from build123d import *

# Parameters (mm, degrees)
F0_R     = 6.35
F1_DEPTH = 12.7
F3_DEPTH = 22.225
F4_W     = 50.8
F4_H     = 25.4
F5_DEPTH = 44.45
F6_R     = 3.175
F7_DEPTH = 25.4


with BuildPart() as f1:
    # F0 (on Front) → F1 (new body)
    with BuildSketch(Plane.XZ):
        with BuildLine():
            Line((64.422844, 12.7), (-62.577156, 12.7))
            ThreePointArc((-62.577156, 12.7), (-75.277156, 0), (-62.577156, -12.7))
            Line((-62.577156, -12.7), (64.422844, -12.7))
            ThreePointArc((64.422844, -12.7), (77.122844, 0), (64.422844, 12.7))
        make_face()
        with Locations((-62.577156, 0)):
            Circle(F0_R, mode=Mode.SUBTRACT)
        with Locations((64.422844, 0)):
            Circle(F0_R, mode=Mode.SUBTRACT)
    extrude(amount=F1_DEPTH)

    # F2 (on Top) → F3 (join, symmetric)
    with BuildSketch(Plane.XY):
        with BuildLine():
            Line((44.45, 0), (-44.45, 0))
            ThreePointArc((-44.45, 0), (0, -44.45), (44.45, 0))
        make_face()
    extrude(amount=F3_DEPTH, both=True)

    # F4 (on face) → F5 (cut)
    with BuildSketch(Plane(origin=(0, 0, -22.225), x_dir=(1, 0, 0), z_dir=(0, 0, -1))):
        with Locations((0, 12.7)):
            Rectangle(F4_W, F4_H)
    extrude(amount=-F5_DEPTH, mode=Mode.SUBTRACT)

    # F6 (on face) → F7 (cut)
    with BuildSketch(Plane(origin=(0, -25.4, 0), x_dir=(-1, 0, 0), z_dir=(0, 1, 0))):
        Circle(F6_R)
    extrude(amount=-F7_DEPTH, mode=Mode.SUBTRACT)


solid = f1.part
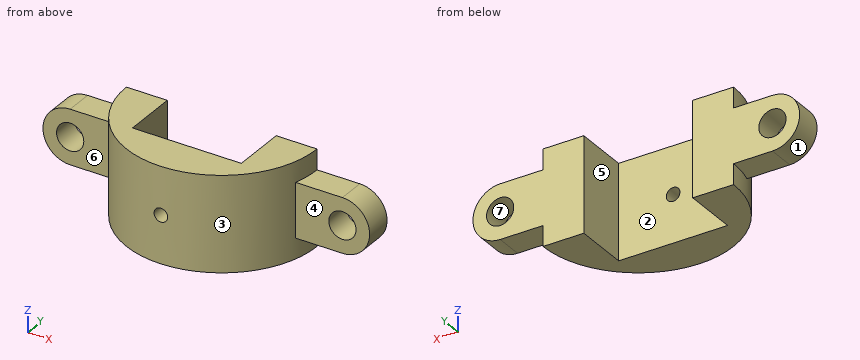
Work out the finished part from the listing and answer in its coordinate system (mm). Face numbers are marked on the shaded views. A direction names the side the tool comes from. Give positions to 0.01 mm unless a question says otherwise; leave off trailing zeros. Loops run counter-clockwise (first coordinate to the right, second up) from the corner with the lowest first, then second, coordinate; pieces in that order, holes last. Notation, with made-up numbers: (15.25, 72) -> (60.25, 72) arc R26 cw to (60.25, 99) -> close; hole circle Ø5 at (76.25, -34). An arc over 180 degrees is marked (long way). Use a Markdown table: item, result. Add a question column.
1) Each of these flat-tipped pins is pushed along its axis until it touches: P1, Ø3, axis at y = -36, z = 15, coming from the -X side; P2, Ø7.5, axis at x = 0, z = 0, coming from the +Y side; P3, Ø7.5, axis at x = 67.5, z = 1, coming from the -Y side. Where does it stop, or does it pass through?
2) The part is cut by section B-B, the plane x = 0. Determine the outline of the cut face in (y, z) (3 decimals).
3) Which of the six approach directions +Z, -Z, +X, -X, +Y, -Y give full straight-line access (tool end or side, diameter ignored) to the marked faces 5, 6 and 7?
4) The part is cut by section C-C, the plane y = -14.5. Determine the outline of the cut face in (x, z) (3 decimals), plus the area to 3 significant figures.
5) Consider line 1 along Z through (x, y) = (0, -39) (3 decimals); line 2 along Y through (x, z) = (71.5, -9.5); line 3 along X through (y, z) = (-16.5, 15). Determine where each line is inside the solid, lowest interval first.
6) The part is cut by section A-A, the plane z = 0. Determine the outline of the cut face in (x, y) (3 decimals).
7) For a pull along X with two mould halves and no side action, classify the marked faces 1, 2, 3 and 4 as +X half, -X half, draft (parallel to the pull), parting line (faces both ways), or undercut.
8) The part is cut by section D-D, the plane y = -5.5. Determine the outline of the cut face in (x, z) (3 decimals).
Reported:
| question | item | result |
|---|---|---|
| 1 | P1 | stops at x = -28.03 |
| 1 | P2 | stops at y = -25.4 |
| 1 | P3 | stops at y = -12.7 |
| 2 | outline | (-44.45, -22.225) -> (-25.4, -22.225) -> (-25.4, -3.175) -> (-44.45, -3.175) -> close; (-44.45, 3.175) -> (-25.4, 3.175) -> (-25.4, 22.225) -> (-44.45, 22.225) -> close |
| 3 | face 5 | +Z, -Z, +Y |
| 3 | face 6 | +Z, -Z, -X, -Y |
| 3 | face 7 | +Y, -Y |
| 4 | outline | (-42.018, -22.225) -> (-25.4, -22.225) -> (-25.4, 22.225) -> (-42.018, 22.225) -> close; (25.4, -22.225) -> (42.018, -22.225) -> (42.018, 22.225) -> (25.4, 22.225) -> close |
| 4 | area | 1,480 mm^2 |
| 5 | line 1 | z = -22.225 to -3.175, 3.175 to 22.225 |
| 5 | line 2 | y = -12.7 to 0 |
| 5 | line 3 | x = -41.27 to -25.4, 25.4 to 41.27 |
| 6 | outline | (-75.277, -12.7) -> (-68.927, -12.7) -> (-68.927, 0) -> (-75.277, 0) -> close; (-56.227, -12.7) -> (-42.597, -12.7) arc R44.45 ccw to (-3.175, -44.336) -> (-3.175, -25.4) -> (-25.4, -25.4) -> (-25.4, 0) -> (-56.227, 0) -> close; (3.175, -44.336) arc R44.45 ccw to (42.597, -12.7) -> (58.073, -12.7) -> (58.073, 0) -> (25.4, 0) -> (25.4, -25.4) -> (3.175, -25.4) -> close; (70.773, -12.7) -> (77.123, -12.7) -> (77.123, 0) -> (70.773, 0) -> close |
| 7 | face 1 | -X half |
| 7 | face 2 | undercut |
| 7 | face 3 | parting line |
| 7 | face 4 | draft |
| 8 | outline | (-62.577, -12.7) -> (-44.108, -12.7) -> (-44.108, -22.225) -> (-25.4, -22.225) -> (-25.4, 22.225) -> (-44.108, 22.225) -> (-44.108, 12.7) -> (-62.577, 12.7) arc R12.7 ccw to start; (25.4, -22.225) -> (44.108, -22.225) -> (44.108, -12.7) -> (64.423, -12.7) arc R12.7 ccw to (64.423, 12.7) -> (44.108, 12.7) -> (44.108, 22.225) -> (25.4, 22.225) -> close; hole circle Ø12.7 at (-62.577, 0); hole circle Ø12.7 at (64.423, 0) |
